Job drawing, mm, ordinate dimensions from the low corner. One solid piece. Round coordinates to 2 decimals unless told otherwise and drop trailing zeros. Loops run counter-clockwise (first coordinate to the right, second up) from the corner with the lowest first, then second, coordinate; pieces in that order, holes last. Notation, with made-up numbers: M -35.5,-29.75 L -31.5,-29.75 A19 ccw -31.5,-4.75 Z; hole C 50,-23.5 d1. An arc over 180 degrees is marked long. Use one line per item in the form item = value.
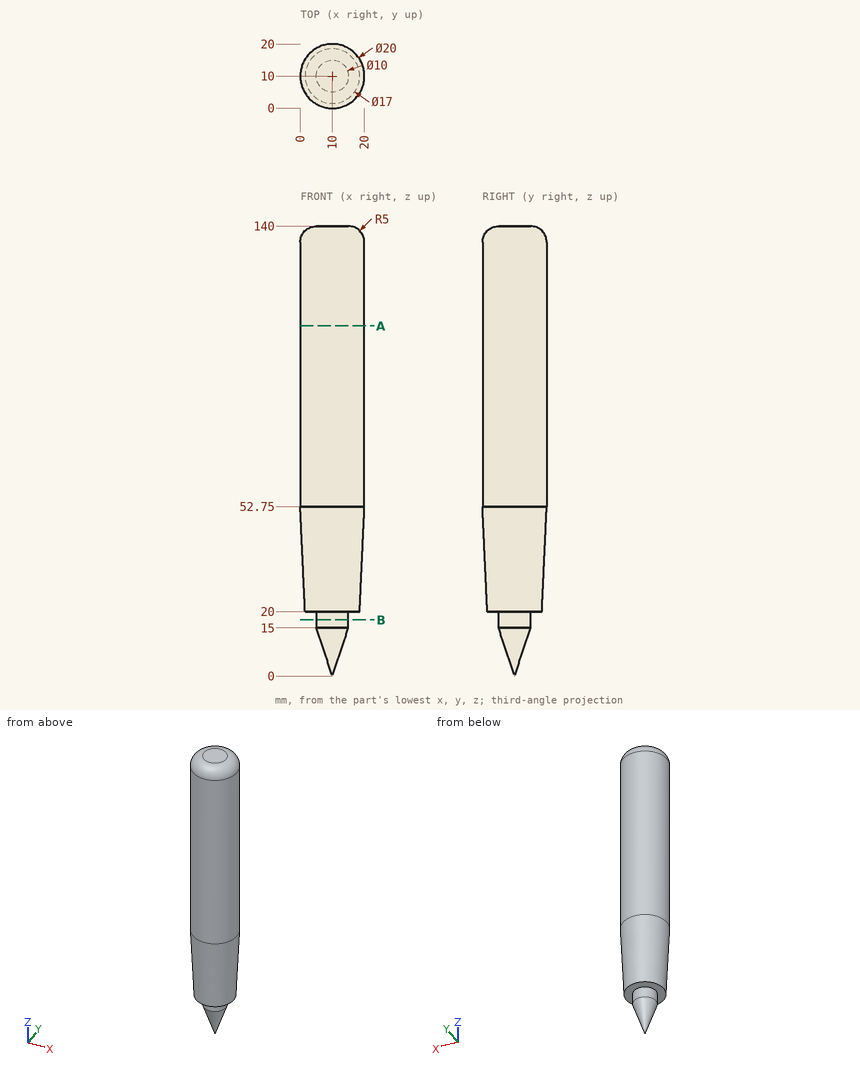
1. Cut at B-B on z = 17.5. Write the cut outline in (x, y).
Completed:
outline = C 10,10 d10
2. Cut at A-A on z = 109. Write the cut outline in (x, y).
Completed:
outline = C 10,10 d20
3. Probe line 1 along Z through (x, y) = (13.25, 14); line 2 along Z through (x, y) = (11.5, 8.5); line 3 along X through (y, z) = (4, 104.5). List the from-to ranges inside material, lowest first. Write a range as from..to.
Completed:
line_1 = 20..140
line_2 = 6.36..140
line_3 = 2..18
4. Drop flat-ended pins along their axis: P1, Ø12, axis at y = 17.5, z = 53, coming from the -X side; P2, Ø3, axis at x = 18, y = 16, coming from the +Z side; P3, Ø5, axis at y = 17, z = 15, coming from the -X side. Give the stop position or say it passes through.
Completed:
P1 = 0.11
P2 = 138.57
P3 = 7.82
